```python
from build123d import *

# Parameters (mm, degrees)
F0_W     = 400
F0_H     = 400
F1_DEPTH = 200
F2_W     = 23.6235832693
F2_H     = 82.5
F2_R     = 8.0037412027
F3_DEPTH = 3
F2_R_2   = 7.7471341156
F4_DEPTH = 3.5
F6_D     = 30
F6_DEPTH = 10
F6_TIP   = 9.0129092854


with BuildPart() as f1:
    # F0 (on Front) → F1 (new body)
    with BuildSketch(Plane.XZ):
        with Locations((138.8336762786, 156.3295841217)):
            Rectangle(F0_W, F0_H)
    extrude(amount=F1_DEPTH)

    # F2 (on face) → F3 (join)
    with BuildSketch(Plane.XZ.offset(200)):
        with Locations((11.8117916346, 135.6753641114)):
            Rectangle(F2_W, F2_H)
        with Locations((11.8117916346, 111.8402481079)):
            Circle(F2_R, mode=Mode.SUBTRACT)
    extrude(amount=F3_DEPTH)

    # F2 (on face) → F4 (join)
    with BuildSketch(Plane.XZ.offset(200)):
        with Locations((11.8117916346, 111.8402481079)):
            Circle(F2_R_2)
    extrude(amount=F4_DEPTH)

    # F6
    with Locations(Plane.XZ.offset(200)):
        with Locations((134.1965198517, 262.6275718212)):
            Hole(F6_D / 2, depth=F6_DEPTH)
            with Locations((0, 0, -(F6_DEPTH + F6_TIP / 2))):  # 118° drill point
                Cone(0, F6_D / 2, F6_TIP, mode=Mode.SUBTRACT)


solid = f1.part
```
Source: CAD feature listing. Evaluate the final solid. Frame: model axes, mm. A direction names the side the tool comes from. Round coordinates to 2 decimals unless told otherwise and drop trailing zeros. Loops run counter-clockwise (first coordinate to the right, second up) from the corner with the lowest first, then second, coordinate; pieces in that order, holes last. Notation, with made-up numbers: M 21,-23.5 L 55,-23.5 A29 cw 55,-3.5 Z; hole C 83.5,84 d5. An arc over 180 degrees is marked long. Use a Markdown table: item, result. Add a question column.
1. Cut plane B-B, the plane x = 177.5. Output: boundary loops of the cut face in (y, z), and give its area (3 significant figures).
2. Ray query, line 1 along Y through (x, z) = (248, 203); line 2 along Y through (x, z) = (5.5, 131). Return the intervals inside material, ascending. Write a range as [from, to].
3. Cut plane A-A, the plane z = 142. Output: boundary loops of the cut face in (x, y).
4. Pull-direction query (X, two-part tool) for faces 1 (the flat face through (12, -203.5, 112)), 2 (the flat face through (338.834, -99, 154)), 3 (the cylindrical face through (10.077, -201.479, 104.027)), 4 (the flat face through (-61.166, -99, 154)); classes: +X half, -X half, draft (parallel to the pull), parting line (faces both ways), or undercut.
5. Contact query for flat-ended pins moving along their axis: pin 1 (8 mm diameter, centred on x = 146, z = 37, fed in from -Y); pin 2 (2.5 mm diameter, centred on x = 10.5, y = -201.5, fed in from -Z); pin 3 (1.5 mm diameter, centred on x = 6.5, y = -201.5, fed in from +Z). Output: stop coordinate, or through.
6. Cut plane C-C, the plane z = 51. Output: boundary loops of the cut face in (x, y), and give its area (3 significant figures).
7. Set-up query: faces 5 (the cylindrical face through (127.275, -194.93, 249.32)), 6 (the flat face through (136, -99, 356.33)). Return all of +Z, -Z, +X, -X, +Y, -Y with unobstructed straight access to the full face (end or side cutting, diameter ignored); none if empty.
Solution:
| question | item | result |
|---|---|---|
| 1 | outline | M -200,-43.67 L 0,-43.67 L 0,356.33 L -200,356.33 Z |
| 1 | area | 80,000 mm2 |
| 2 | line 1 | y = [-200, 0] |
| 2 | line 2 | y = [-203, 0] |
| 3 | outline | M -61.17,-200 L 0,-200 L 0,-203 L 23.62,-203 L 23.62,-200 L 338.83,-200 L 338.83,0 L -61.17,0 Z |
| 4 | face 1 | draft |
| 4 | face 2 | +X half |
| 4 | face 3 | undercut |
| 4 | face 4 | -X half |
| 5 | pin 1 | stops at y = -200 |
| 5 | pin 2 | stops at z = 94.43 |
| 5 | pin 3 | stops at z = 176.93 |
| 6 | outline | M -61.17,-200 L 338.83,-200 L 338.83,0 L -61.17,0 Z |
| 6 | area | 80,000 mm2 |
| 7 | face 5 | -Y |
| 7 | face 6 | +Z, +X, -X, +Y, -Y |
